Work out the finished part from the listing and answer in its coordinate system (mm). A direction names the side the tool comes from. Coordinates: 2 decimals unless noted, no trailing zeros. Order: outer loops, then holes, each group sorted by start corner. A loop starts at its lowest first (then second) coordinate and runs counter-clockwise, first axis right, second up. Notation, with made-up numbers: M 3.25,86 L 50.25,86 A21 ccw 50.25,96 Z; hole C 75,-2.5 d4. An arc over 180 degrees is marked long. Use a Markdown table: item, result. Add a question column.
Autodesk Inventor part; units mm, degrees
ref_plane "YZ Plane" through (0, 0, 0) normal (1, 0, 0) x (0, 1, 0)
ref_plane "XZ Plane" through (0, 0, 0) normal (0, 1, 0) x (-1, 0, 0)
ref_plane "XY Plane" through (0, 0, 0) normal (0, 0, 1) x (1, 0, 0)
sketch "Sketch1" plane through (0, 0, 0) normal (0, 0, 1) x (1, 0, 0)
  line L0 (0, 0) -> (-3.175, 0)
  line L1 (-3.175, 0) -> (-3.175, -384.175)
  line L2 (-3.175, -384.175) -> (0, -384.175)
  line L3 (0, -384.175) -> (0, 0)
  dimension "d0" = 3.175
  dimension "d1" = 384.175
extrude "Extrusion1" add sketch "Sketch1" along normal blind 152.4
sketch "Sketch2" plane through (-3.175, -384.175, 0) normal (-1, 0, 0) x (0, 0, 1)
  line L0 (0, 384.175) -> (0, 0)
  line L1 (152.4, 384.175) -> (0, 384.175)
  line L2 (0, 384.175) -> (0, 381)
  line L3 (0, 381) -> (152.4, 381)
  line L4 (152.4, 381) -> (152.4, 384.175)
  line L5 (0, 384.175) -> (152.4, 384.175)
  line L6 (152.4, 384.175) -> (152.4, 0)
  line L7 (152.4, 0) -> (0, 0)
  line L8 (0, 0) -> (0, 3.175)
  line L9 (0, 3.175) -> (152.4, 3.175)
  line L10 (152.4, 3.175) -> (152.4, 0)
  dimension "d4" = 152.4
  dimension "d5" = 3.175
  dimension "d6" = 3.175
extrude "Extrusion2" add sketch "Sketch2" along normal blind 152.4 contours L1 L4 L3 L0 | L9 L6 L7 L0
sketch "Sketch3" plane through (0, -384.175, 0) normal (0, -1, 0) x (1, 0, 0)
  line L0 (-3.175, 152.4) -> (49.7899, 295.3003)
  line L1 (49.7899, 295.3003) -> (52.767, 294.1968)
  line L2 (52.767, 294.1968) -> (-0.1979, 151.2966)
  line L3 (-0.1979, 151.2966) -> (-3.175, 152.4)
  point P0 (0, 0)
  dimension "d9" = 3.175
  dimension "d10" = 152.4
extrude "Extrusion3" add sketch "Sketch3" against normal blind 384.175
(1) Straight lines are drawn through the part: line 1 (Y direction, x = -66.5, z = 119) (3 decimals); line 2 (X direction, y = -131, z = 136.5) (3 decimals); line 3 (X direction, y = -100.5, z = 240.5). For each, find the intervals that lie inside material, in ascending order.
(2) Which of the six approach directions +Z, -Z, +X, -X, +Y, -Y give full straight-line access (tool end or side, diameter ignored) to faces 1 (the flat face through (-78, -3.175, 75)), 2 (the flat face through (-76, -384.175, 84)), 3 (the flat face through (0, -195, 75))?
(3) A cutting plane is placed at A-A on x = -49.5. Write down the section's boundary in (y, z) (3 decimals), plus the area to 3 significant figures.
(4) The mould has two halves that part along Y. Classify faces 4 (the flat face through (-78, -381, 75)), 5 (the flat face through (-76, 0, 84)), 6 (the flat face through (-3.175, -189, 75)), 7 (the flat face through (22.937, -194.777, 222.85)): pulls with the +Y half, pulls with the -Y half, needs draft (parallel to the pull), parting line crosses it, or undercut.
(5) Given P1, Ø8, axis at y = -323.5, z = 182.5, coming from the +X side; P2, Ø1, axis at x = -53, y = -383, coming from the +Z side; P3, Ø6, axis at y = -44.5, z = 117.5, coming from the +X side, each flat-ended and moving along its own axis, determine where each tip first touches the part or whether it passes through.
(6) A cutting plane is placed at C-C on y = -103. Write down the section's boundary in (x, z) (3 decimals).
(7) A cutting plane is placed at D-D on x = 25. Write down the section's boundary in (y, z) (3 decimals).
(8) A cutting plane is placed at B-B on z = 120. Write down the section's boundary in (x, y) (3 decimals), plus the area to 3 significant figures.
From the geometry:
| question | item | result |
|---|---|---|
| 1 | line 1 | y = -384.175 to -381, -3.175 to 0 |
| 1 | line 2 | x = -3.175 to 0 |
| 1 | line 3 | x = 29.48 to 32.86 |
| 2 | face 1 | +Z, -Z, -X |
| 2 | face 2 | +Z, -Z, +X, -X, -Y |
| 2 | face 3 | -Z, +X, +Y, -Y |
| 3 | outline | M -384.175,0 L -381,0 L -381,152.4 L -384.175,152.4 Z; M -3.175,0 L 0,0 L 0,152.4 L -3.175,152.4 Z |
| 3 | area | 968 mm2 |
| 4 | face 4 | undercut |
| 4 | face 5 | pulls with the +Y half |
| 4 | face 6 | undercut |
| 4 | face 7 | needs draft |
| 5 | P1 | stops at x = 12.85 |
| 5 | P2 | stops at z = 152.4 |
| 5 | P3 | stops at x = 0 |
| 6 | outline | M -3.175,0 L 0,0 L 0,151.831 L 52.767,294.197 L 49.79,295.3 L -3.175,152.4 Z |
| 7 | outline | M -384.175,219.281 L 0,219.281 L 0,228.417 L -384.175,228.417 Z |
| 8 | outline | M -155.575,-384.175 L 0,-384.175 L 0,0 L -155.575,0 L -155.575,-3.175 L -3.175,-3.175 L -3.175,-381 L -155.575,-381 Z |
| 8 | area | 2,190 mm2 |
